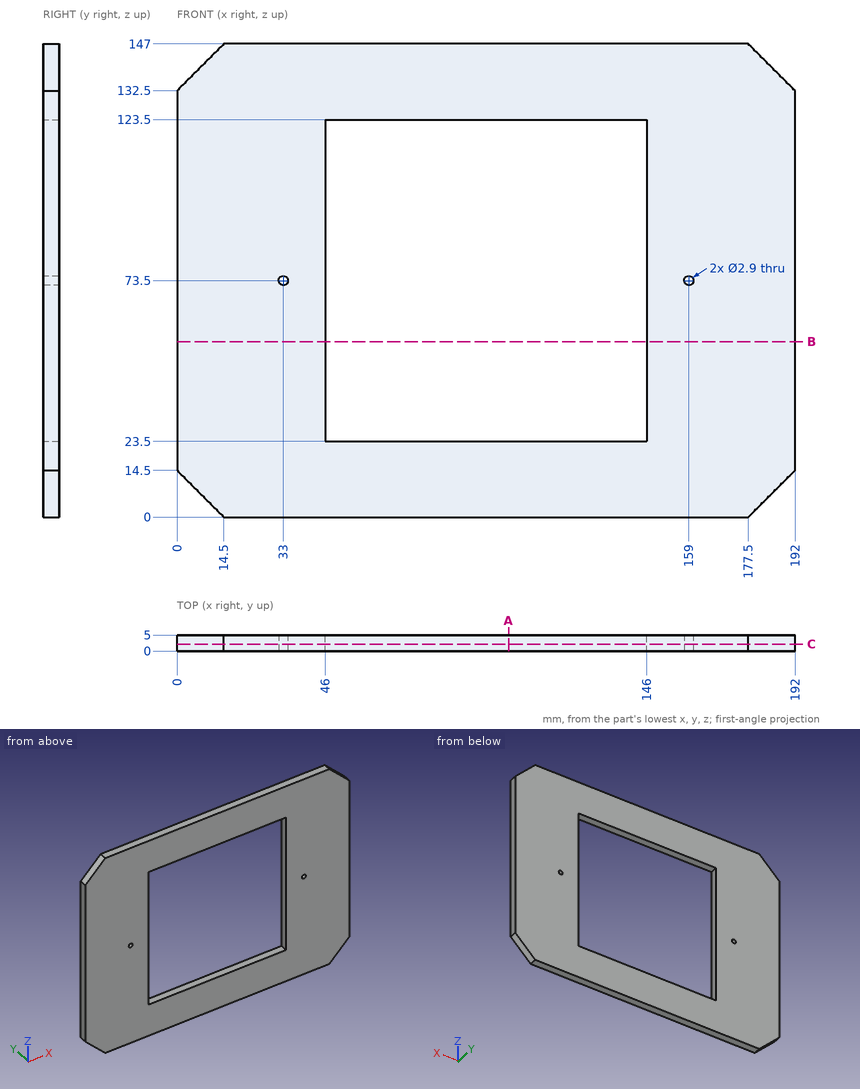
Geometry: see drawing. Coordinates: mm, zero at the bounding-box minimum. Round coordinates to 2 decimals unless told otherwise and drop trailing zeros. Write each loop counter-clockwise with the first axis right and the second up, starting at its lowest first coordinate (ties: lowest second). Pieces come first, ordered by that corner, then holes.
1) Cut plane C-C (y = 2.2). Return the cut outline in (x, z), then the cut area to 3 significant figures.
2) Cut plane A-A (x = 103). Return the cut outline in (y, z).
3) Cut plane B-B (z = 54.5). Return the cut outline in (x, y).
4) Ray query, L1, parallel to X at y = 2, z = 73.5; L2, parallel to X at y = 1.2, z = 89; L3, parallel to Z at x = 90, y = 4.45. Return the intervals inside material, ascending.
Geometry says:
1. outline: (0, 14.5) - (14.5, 0) - (177.5, 0) - (192, 14.5) - (192, 132.5) - (177.5, 147) - (14.5, 147) - (0, 132.5) - close; hole circle Ø2.9 at (33, 73.5); hole (46, 23.5) - (146, 23.5) - (146, 123.5) - (46, 123.5) - close; hole circle Ø2.9 at (159, 73.5)
1. area: 17,800 mm2
2. outline: (0, 0) - (5, 0) - (5, 23.5) - (0, 23.5) - close; (0, 123.5) - (5, 123.5) - (5, 147) - (0, 147) - close
3. outline: (0, 0) - (46, 0) - (46, 5) - (0, 5) - close; (146, 0) - (192, 0) - (192, 5) - (146, 5) - close
4. L1: x = 0 to 31.55, 34.45 to 46, 146 to 157.55, 160.45 to 192
4. L2: x = 0 to 46, 146 to 192
4. L3: z = 0 to 23.5, 123.5 to 147
